Source: CAD feature listing. Evaluate the final solid. Frame: model axes, mm. A direction names the side the tool comes from. Give positions to 0.01 mm unless a question says otherwise; leave off trailing zeros. Write each loop counter-clockwise with the first axis right and the second up, starting at its lowest first coordinate (ties: lowest second). Pieces come first, ordered by that corner, then holes. Notation, with made-up numbers: (-15, -4) -> (-1, -4) arc R23 ccw to (-1, 7) -> close; hole circle Ø6 at (83, -31). An arc over 180 degrees is marked (long way). Answer as a JSON object with one key per item and string values. Group by question number.
Item 1: Section query D-D on z = 3.5. Give the number of separate pieces and of enclosed holes in the cut face, plus the area to 3 significant figures.
Item 2: First-contact query: pin 1 Ø3 at (x, z) = (61.5, -3.5) entering from -Y; pin 2 Ø8 at (x, y) = (0, -75) entering from -Z; pin 3 Ø1 at (y, z) = (13, 3) entering from +X. Flat tips, straight axial feed; report the tip coordinate or a pass-through.
Item 3: Access query for faces 3 (the face through (53.301, 64.705, 2.465)), 4 (the face through (-28, -21, 2)), 5 (the face through (-75.04, -36.99, -2.46)). Directions: +Z, -Z, +X, -X, +Y, -Y. A direction counts if a zero-diameter tool reaches every point of the face in a straight line with its end or side. Return the directions, or none.
Item 4: Section query A-A on x = 0. Return the cut outline in (y, z), plus the area to 3 significant figures.
Item 5: Ray query, probe 1 along Y at (x, z) = (0, 1.8); probe 2 along Y at (x, z) = (-77, 0.25); probe 3 along Z at (x, y) = (-58, -2). Return the intervals inside material, ascending. Write a range as from..to.
Item 6: Pull-direction query (X, two-part tool) for faces 1 (the face through (55, 71, -5)), 2 (the face through (-83, -35, 0)); classes: pulls with the +X half, pulls with the -X half, needs draft (parallel to the pull), parting line crosses it, or undercut.
Item 7: Section query C-C on y = 75. Return the cut outline in (x, z), plus the area to 3 significant figures.
Item 8: Section query B-B on y = 0. Return the cut outline in (x, z), plus the area to 3 significant figures.
from build123d import *

# Parameters (mm, degrees)
F0_R     = 2.5
F0_R_2   = 6.86
F0_R_3   = 35
F1_DEPTH = 5
F2_R     = 8.5
F3_DEPTH = 5


with BuildPart() as f1:
    # F0 (on Top) → F1 (new body)
    with BuildSketch(Plane.XY):
        with BuildLine():
            Line((57.236352, 82), (-57.236352, 82))
            ThreePointArc((-57.236352, 82), (0, -100), (57.236352, 82))
        make_face()
        with Locations((0, -75)):
            Circle(F0_R, mode=Mode.SUBTRACT)
        with Locations((-83.149158, -34.441509)):
            Circle(F0_R_2, mode=Mode.SUBTRACT)
        with Locations((83.149158, -34.441509)):
            Circle(F0_R_2, mode=Mode.SUBTRACT)
        with Locations((-75, 0)):
            Circle(F0_R, mode=Mode.SUBTRACT)
        Circle(F0_R_3, mode=Mode.SUBTRACT)
        with Locations((-54.788529, 71.401801)):
            Circle(F0_R_2, mode=Mode.SUBTRACT)
        with Locations((0, 75)):
            Circle(F0_R, mode=Mode.SUBTRACT)
        with Locations((75, 0)):
            Circle(F0_R, mode=Mode.SUBTRACT)
        with Locations((54.788529, 71.401801)):
            Circle(F0_R_2, mode=Mode.SUBTRACT)
    extrude(amount=F1_DEPTH)

    # F2 (on face) → F3 (join)
    with BuildSketch(Plane(origin=(0, 0, 0), x_dir=(1, 0, 0), z_dir=(0, 0, -1))):
        with Locations((83.149158, 34.441509)):
            Circle(F2_R)
        with Locations((54.788529, -71.401801)):
            Circle(F2_R)
        with Locations((-54.788529, -71.401801)):
            Circle(F2_R)
        with Locations((-83.149158, 34.441509)):
            Circle(F2_R)
    extrude(amount=F3_DEPTH)


solid = f1.part
Worked answers:
{
 "1": {"separate pieces": "1", "enclosed holes": "9", "area": "25,500 mm^2"},
 "2": {"pin 1": "y = 64.69", "pin 2": "z = 0", "pin 3": "x = 99.22"},
 "3": {"face 3": "+Z", "face 4": "+Z, -Z", "face 5": "-Z"},
 "4": {"outline": "(-100, 0) -> (-77.5, 0) -> (-77.5, 5) -> (-100, 5) -> close; (-72.5, 0) -> (-35, 0) -> (-35, 5) -> (-72.5, 5) -> close; (35, 0) -> (72.5, 0) -> (72.5, 5) -> (35, 5) -> close; (77.5, 0) -> (82, 0) -> (82, 5) -> (77.5, 5) -> close", "area": "510 mm^2"},
 "5": {"probe 1": "-100..-77.5, -72.5..-35, 35..72.5, 77.5..82", "probe 2": "-63.8..-37.48, -31.4..-1.5, 1.5..63.8", "probe 3": "0..5"},
 "6": {"face 1": "needs draft", "face 2": "undercut"},
 "7": {"outline": "(-66.14, 0) -> (-62.49, 0) -> (-62.49, -5) -> (-47.09, -5) -> (-47.09, 0) -> (-2.5, 0) -> (-2.5, 5) -> (-48.95, 5) -> (-48.95, 0) -> (-60.63, 0) -> (-60.63, 5) -> (-66.14, 5) -> close; (2.5, 0) -> (47.09, 0) -> (47.09, -5) -> (62.49, -5) -> (62.49, 0) -> (66.14, 0) -> (66.14, 5) -> (60.63, 5) -> (60.63, 0) -> (48.95, 0) -> (48.95, 5) -> (2.5, 5) -> close", "area": "674 mm^2"},
 "8": {"outline": "(-100, 0) -> (-77.5, 0) -> (-77.5, 5) -> (-100, 5) -> close; (-72.5, 0) -> (-35, 0) -> (-35, 5) -> (-72.5, 5) -> close; (35, 0) -> (72.5, 0) -> (72.5, 5) -> (35, 5) -> close; (77.5, 0) -> (100, 0) -> (100, 5) -> (77.5, 5) -> close", "area": "600 mm^2"}
}
